from build123d import *

# Parameters (mm, degrees)
F0_R          = 14.2875
F0_R_2        = 12.7
F2_DEPTH      = 50.8
F3_R          = 26.9875
F3_R_2        = 14.2875
F4_DEPTH      = 63.5
F4_DEPTH_BACK = 12.7
F5_SIZE       = 7.62
F7_START      = -26.67
F6_W          = 64.1522035003
F6_H          = 10.4847997427
F7_DEPTH      = 6.35
F8_R          = 1.26999


# Not quite as in the source:
# - a fillet or chamfer is up to 0.001 mm smaller than in the source, because OpenCascade refuses the exact size
# - a feature names something its author has since deleted; it is built from what else it names


with BuildPart() as f2:
    # F0 (on Top) → F2 (new body)
    with BuildSketch(Plane.XY):
        Circle(F0_R)
        Circle(F0_R_2, mode=Mode.SUBTRACT)
    extrude(amount=F2_DEPTH)

    # F3 (on face) → F4 (join, two sides)
    with BuildSketch(Plane.XY) as f4_sk:
        Circle(F3_R)
        Circle(F3_R_2, mode=Mode.SUBTRACT)
    extrude(amount=F4_DEPTH)
    extrude(f4_sk.sketch, amount=-F4_DEPTH_BACK)

    # F5
    f5_edges = [f2.edges().sort_by_distance(p)[0] for p in [
        (-26.9875, 0, 63.5),
        (-26.9875, 0, -12.7),
    ]]
    chamfer(f5_edges, length=F5_SIZE)

    # F6 (on Front) → F7 (join)
    with BuildSketch(Plane.XZ.offset(F7_START)):
        with Locations((23.3749561012, 26.5372619033)):
            Rectangle(F6_W, F6_H)
    extrude(amount=-F7_DEPTH)

    # F8 (radius 1.27 in the source; OpenCascade refuses exactly that, so slightly less here)
    f8_edges = [f2.edges().sort_by_distance(p)[0] for p in [
        (23.374956, 33.02, 31.779662),
        (23.374956, 33.02, 21.294862),
        (-8.701146, 33.02, 26.537262),
        (29.789279, 26.67, 21.294862),
        (29.789279, 26.67, 31.779662),
        (55.451058, 26.67, 26.537262),
        (55.451058, 29.845, 31.779662),
        (55.451058, 33.02, 26.537262),
        (55.451058, 29.845, 21.294862),
    ]]
    fillet(f8_edges, radius=F8_R)


solid = f2.part
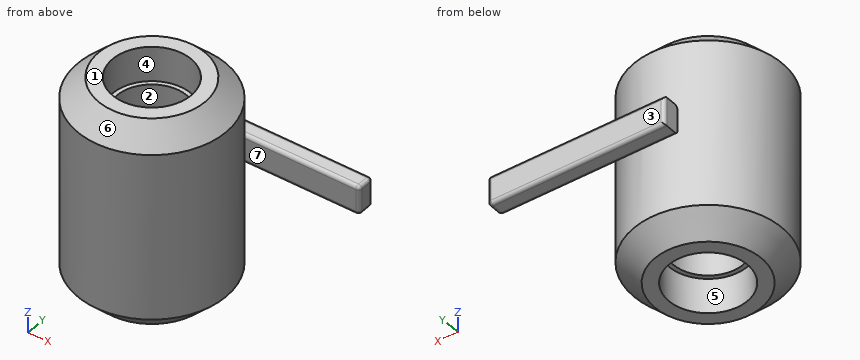
Read the model definition and answer for the solid it produces. Units are mm, in the model's axes. Face numbers are marked on the shaded views. A direction names the side the tool comes from. Round coordinates to 2 decimals unless told otherwise and drop trailing zeros. Order: outer loops, then holes, each group sorted by start corner. A loop starts at its lowest first (then second) coordinate and runs counter-clockwise, first axis right, second up. Notation, with made-up numbers: (-27, 7.25) - (-17, 7.25) arc R26 ccw to (-17, 46.25) - close; hole circle Ø10 at (-24.5, 12.5). An arc over 180 degrees is marked (long way). Use one line per item in the form item = value. Start each with the question number.
(1) For the marked faces 5, 6 and 7, determine the directions among +Z, -Z, +X, -X, +Y, -Y from which every point of the face is accessible in a straight line to the end or side of a thin tool.
(2) The part is cut by section C-C (x = 33.5). Give the vertices of the cut face in (y, z).
(3) The part is cut by section D-D (z = 3.5). Give the vertices of the cut face in (x, y) (1 decimal), then the cut area to 3 significant figures.
(4) Flat-ended cylindrical pins translate along their axes: pin 1 Ø6.5 at (x, z) = (31, 26.5) entering from -Y; pin 2 Ø4 at (x, z) = (23.5, 15) entering from +Y; pin 3 Ø5 at (x, y) = (3, -9) entering from -Z; pin 4 Ø12 at (x, y) = (26.5, 0.5) entering from +Z. Find the tip coordinate at first contact, or state that the pin passes through.
(5) The part is cut by section A-A (y = 0). Give the vertices of the cut face in (x, z).
(6) Determine the mould class of the marked faces 1, 2, 3 and 4 for opening direction Y: +Y half, -Y half, draft (parallel to the pull), parting line (faces both ways), or undercut.
(7) The part is cut by section B-B (x = 0). Give the vertices of the cut face in (y, z).
(8) Find the intervals of material crossed by line 1 along Y through (x, z) = (45, 24.5); line 2 along Y through (x, z) = (0, 58.25); line 3 along X through (y, z) = (6.5, 44), in increasing order. Write a range as from..to.
Checked values:
q1.face_5 = -Z
q1.face_6 = +Z
q1.face_7 = +Z, -Z, +X
q2.outline = (26.67, 22.56) arc R1.27 ccw to (27.94, 21.29) - (31.75, 21.29) arc R1.27 ccw to (33.02, 22.56) - (33.02, 30.51) arc R1.27 ccw to (31.75, 31.78) - (27.94, 31.78) arc R1.27 ccw to (26.67, 30.51) - close
q3.outline = circle Ø54 at (0, 0); hole circle Ø25.4 at (0, 0)
q3.area = 1,780 mm^2
q4.pin_1 = 26.67
q4.pin_2 = 16.31
q4.pin_3 = through
q4.pin_4 = 62.36
q5.outline = (-26.99, -5.08) - (-19.37, -12.7) - (-14.29, -12.7) - (-14.29, 0) - (-12.7, 0) - (-12.7, 50.8) - (-14.29, 50.8) - (-14.29, 63.5) - (-19.37, 63.5) - (-26.99, 55.88) - close; (12.7, 0) - (14.29, 0) - (14.29, -12.7) - (19.37, -12.7) - (26.99, -5.08) - (26.99, 55.88) - (19.37, 63.5) - (14.29, 63.5) - (14.29, 50.8) - (12.7, 50.8) - close
q6.face_1 = draft
q6.face_2 = undercut
q6.face_3 = +Y half
q6.face_4 = undercut
q7.outline = (-26.99, -5.08) - (-19.37, -12.7) - (-14.29, -12.7) - (-14.29, 0) - (-12.7, 0) - (-12.7, 50.8) - (-14.29, 50.8) - (-14.29, 63.5) - (-19.37, 63.5) - (-26.99, 55.88) - close; (12.7, 0) - (14.29, 0) - (14.29, -12.7) - (19.37, -12.7) - (26.99, -5.08) - (26.99, 21.72) arc R1.27 ccw to (27.94, 21.29) - (31.75, 21.29) arc R1.27 ccw to (33.02, 22.56) - (33.02, 30.51) arc R1.27 ccw to (31.75, 31.78) - (27.94, 31.78) arc R1.27 ccw to (26.99, 31.35) - (26.99, 55.88) - (19.37, 63.5) - (14.29, 63.5) - (14.29, 50.8) - (12.7, 50.8) - close
q8.line_1 = 26.67..33.02
q8.line_2 = -24.62..-14.29, 14.29..24.62
q8.line_3 = -26.19..-10.91, 10.91..26.19
